Part model, mm, in its own coordinate system. A direction names the side the tool comes from. Give positions to 0.01 mm unless a question says otherwise; leave off trailing zeros. Order: outer loops, then holes, each group sorted by start corner. A loop starts at its lowest first (then second) coordinate and runs counter-clockwise, first axis right, second up.
1. Drop flat-ended pins along their axis: pin 1 Ø0.7 at (y, z) = (4, -9) entering from +X; pin 2 Ø5.5 at (x, y) = (-67.5, 11) entering from +Z; pin 3 Ø1 at (x, y) = (7.5, 4.5) entering from -Z (3 decimals). Give the stop position or say it passes through.
2. Which spindle directions (+Z, -Z, +X, -X, +Y, -Y) get a long thin tool onto all of the face, cutting with end or side? Do faces 1 (the flat face through (0, 7.62, -7)), 2 (the flat face through (-21, -2, -10)), 3 (the flat face through (-59.454, 9, -18)). Say none if no direction does.
3. Slice it at C-C on z = -1.5. List the corners of the cut face in (x, y).
4. Mould opens along X. For faces 4 (the flat face through (-7.714, 4, -4)), 5 (the cylindrical face through (-61.63, 13.42, -2.08)), 6 (the flat face through (-7.714, 4, 4)), 7 (the cylindrical face through (-65.533, 5.59, -10.656)) say: +X half, -X half, draft (parallel to the pull), parting line (faces both ways), or undercut.
5. Slice it at D-D on z = -23. List the corners of the cut face in (x, y), and give its area (3 significant figures).
6. Probe line 1 (X direction, y = -3, z = 0); line 2 (Z direction, x = -67.75, y = 6.35); line 3 (X direction, y = 3.75, z = 1.5). List the from-to ranges inside material, lowest first.
7. Slice it at A-A on x = 0. List the corners of the cut face in (y, z), and give its area (3 significant figures).
8. Slice it at B-B on y = 15.5. List the corners of the cut face in (x, z), and give its area (3 significant figures).
from build123d import *

# Parameters (mm, degrees)
BOSS_EXTRUDE1_DEPTH   = 7.62
BOSS_EXTRUDE1_2_DEPTH = 7.62
BOSS_EXTRUDE1_3_DEPTH = 7.62
BOSS_EXTRUDE1_4_DEPTH = 7.62
SKETCH2_W             = 82.1538108
SKETCH2_H             = 20
BOSS_EXTRUDE2_DEPTH   = 6.35
CUT_EXTRUDE1_DEPTH    = 75.17097352
FILLET1_R             = 2.54
SKETCH6_W             = 25.4
SKETCH6_H             = 25.4
BOSS_EXTRUDE7_DEPTH   = 12.7
FILLET3_R             = 7.62
FILLET5_R             = 7.62
SKETCH11_R            = 1.984375
CUT_EXTRUDE3_DEPTH    = 89.015038158
SKETCH12_R            = 3.556
CUT_EXTRUDE4_DEPTH    = 79.762749597


with BuildPart() as part:
    # Sketch1 → Boss-Extrude1 (new body)
    with BuildSketch(Plane(origin=(0, 0, 0), x_dir=(1, 0, 0), z_dir=(0, 1, 0))):
        Polygon((-2.9718, 10), (-2.9718, 7.714), (-4.4450054, 7.714), (-4.4450054, 6.444), (-2.9718, 4.158), (2.9718, 4.158), (4.4449946, 6.444), (4.4449946, 7.714), (2.9718, 7.714), (2.9718, 10), align=None)
    extrude(amount=BOSS_EXTRUDE1_DEPTH)



with BuildPart() as body_2:
    # Sketch1 → Boss-Extrude1 2 (new body)
    with BuildSketch(Plane(origin=(0, 0, 0), x_dir=(1, 0, 0), z_dir=(0, 1, 0))):
        Polygon((4.158, -2.9718), (4.158, 2.9718), (6.444, 4.4449946), (7.714, 4.4449946), (7.714, 2.9718), (10, 2.9718), (10, -2.9718), (7.714, -2.9718), (7.714, -4.4450054), (6.444, -4.4450054), align=None)
    extrude(amount=BOSS_EXTRUDE1_2_DEPTH)


with BuildPart() as body_3:
    # Sketch1 → Boss-Extrude1 3 (new body)
    with BuildSketch(Plane(origin=(0, 0, 0), x_dir=(1, 0, 0), z_dir=(0, 1, 0))):
        Polygon((4.4450054, -6.444), (2.9718, -4.158), (-2.9718, -4.158), (-4.4449946, -6.444), (-4.4449946, -7.714), (-2.9718, -7.714), (-2.9718, -10), (2.9718, -10), (2.9718, -7.714), (4.4450054, -7.714), align=None)
    extrude(amount=BOSS_EXTRUDE1_3_DEPTH)


with BuildPart() as body_4:
    # Sketch1 → Boss-Extrude1 4 (new body)
    with BuildSketch(Plane(origin=(0, 0, 0), x_dir=(1, 0, 0), z_dir=(0, 1, 0))):
        Polygon((-10, -2.9718), (-10, 2.9718), (-7.714, 2.9718), (-7.714, 4.4450054), (-6.444, 4.4450054), (-4.158, 2.9718), (-4.158, -2.9718), (-6.444, -4.4449946), (-7.714, -4.4449946), (-7.714, -2.9718), align=None)
    extrude(amount=BOSS_EXTRUDE1_4_DEPTH)


with BuildPart() as part_1:
    add(part.part)

    add(body_2.part)  # Boss-Extrude2 merges body 2

    add(body_3.part)  # Boss-Extrude2 merges body 3

    add(body_4.part)  # Boss-Extrude2 merges body 4
    # Sketch2 → Boss-Extrude2 (add)
    with BuildSketch(Plane.XZ):
        with Locations((-31.0769054, 0)):
            Rectangle(SKETCH2_W, SKETCH2_H)
    extrude(amount=BOSS_EXTRUDE2_DEPTH)

    # Sketch4 → Cut-Extrude1 (cut, through all)
    with BuildSketch(Plane(origin=(0, -6.35, 0), x_dir=(-1, 0, 0), z_dir=(0, -1, 0))):
        Polygon((72.1538108, -10), (34.6126108, -10), (72.1538108, -0.2108), align=None)
    extrude(amount=-CUT_EXTRUDE1_DEPTH, mode=Mode.SUBTRACT)

    # Fillet1
    fillet1_edges = [part_1.edges().sort_by_distance(p)[0] for p in [
        (-34.6126108, -3.175, 10),
    ]]
    fillet(fillet1_edges, radius=FILLET1_R)

    # Sketch6 → Boss-Extrude7 (add)
    with BuildSketch(Plane.ZY.offset(72.1538108)):
        with Locations((-12.4892, 6.35)):
            Rectangle(SKETCH6_W, SKETCH6_H)
    extrude(amount=-BOSS_EXTRUDE7_DEPTH)

    # Fillet3
    fillet3_edges = [part_1.edges().sort_by_distance(p)[0] for p in [
        (-59.4538108, 0, -4.8946),
        (-59.4538108, -3.175, -10),
    ]]
    fillet(fillet3_edges, radius=FILLET3_R)

    # Fillet5
    # the kernel refuses this fillet: 7.62 mm, written as the material it takes off along each edge
    with BuildSketch(Plane(origin=(-59.4538108, 38.1, 0.2108), x_dir=(-1, 0, 0), z_dir=(0, -1, 0))) as fillet5_piece_1:
        with BuildLine():
            CenterArc((FILLET5_R, FILLET5_R), FILLET5_R, 180, 90)
            Line((0, FILLET5_R), (0, 0))
            Line((0, 0), (FILLET5_R, 0))
        make_face()
    extrude(amount=30.48, mode=Mode.SUBTRACT)
    with BuildSketch(Plane(origin=(-51.8338108, 7.62, 0.2108), x_dir=(0.5976672776328273, 0.8017442392976484, 0), z_dir=(-0.8017442392976484, 0.5976672776328273, 0))) as fillet5_piece_2_section:
        with BuildLine():
            CenterArc((7.62 + FILLET5_R, FILLET5_R), FILLET5_R, 180, 90)
            Line((7.62, FILLET5_R), (7.62, 0))
            Line((7.62, 0), (7.62 + FILLET5_R, 0))
        make_face()
    fillet5_piece_2 = revolve(axis=Axis((-51.8338108, 7.62, 0.2108), (0, 0, -1)), revolution_arc=233.296989237, mode=Mode.PRIVATE)
    fillet5_piece_2 = split(fillet5_piece_2, bisect_by=Plane(origin=(-57.548345525, 0, -2.163807672), z_dir=(0, 1, 0)), keep=Keep.TOP, mode=Mode.PRIVATE)
    add(fillet5_piece_2, mode=Mode.SUBTRACT)

    # Sketch11 → Cut-Extrude3 (cut, through all)
    with BuildSketch(Plane.ZY.offset(72.1538108)):
        with Locations((-12.4892, 6.35)):
            Circle(SKETCH11_R)
    extrude(amount=-CUT_EXTRUDE3_DEPTH, mode=Mode.SUBTRACT)

    # Sketch12 → Cut-Extrude4 (cut, through all)
    with BuildSketch(Plane(origin=(0, 0, 0), x_dir=(1, 0, 0), z_dir=(0, 1, 0))):
        with Locations(Location((0, 0, 0), (0, 0, 270))):
            Circle(SKETCH12_R)
    extrude(amount=-CUT_EXTRUDE4_DEPTH, mode=Mode.SUBTRACT)


solid = part_1.part
Data:
1. pin 1: stops at x = 2.97
1. pin 2: stops at z = 0.21
1. pin 3: stops at z = -4.445
2. face 1: +Z, -Z, +X, +Y
2. face 2: -Z, +X, +Y, -Y
2. face 3: -Z, +X, +Y
3. outline: (-72.15, -6.35) - (-3.22, -6.35) - (-3.22, 0) - (-4.16, 0) - (-4.16, 7.62) - (-10, 7.62) - (-10, 0) - (-58.95, 0) arc R10.43 cw to (-62.26, 7.62) - (-62.26, 19.05) - (-72.15, 19.05) - close; (3.22, -6.35) - (10, -6.35) - (10, 7.62) - (4.16, 7.62) - (4.16, 0) - (3.22, 0) - close
4. face 4: undercut
4. face 5: +X half
4. face 6: -X half
4. face 7: draft
5. outline: (-72.15, -6.35) - (-59.45, -6.35) - (-59.45, 19.05) - (-72.15, 19.05) - close
5. area: 323 mm2
6. line 1: x = -72.15 to -3.56, 3.56 to 10
6. line 2: z = -25.19 to -14.47, -10.5 to 0.21
6. line 3: x = -10 to -4.16, 4.16 to 10
7. outline: (-6.35, -10) - (7.62, -10) - (7.62, -4.16) - (0, -4.16) - (0, -3.56) - (-6.35, -3.56) - close; (-6.35, 3.56) - (0, 3.56) - (0, 4.16) - (7.62, 4.16) - (7.62, 10) - (-6.35, 10) - close
7. area: 171 mm2
8. outline: (-72.15, -25.19) - (-59.45, -25.19) - (-59.45, -7.41) arc R7.62 ccw to (-67.07, 0.21) - (-72.15, 0.21) - close
8. area: 310 mm2
